Design review of the part built by this model. Coordinates are the model's own, in mm. Face numbers are marked on the shaded views. A direction names the side the tool comes from. Give positions to 0.01 mm unless a question says otherwise; leave off trailing zeros. Order: outer loops, then holes, each group sorted by start corner. A loop starts at its lowest first (then second) coordinate and runs counter-clockwise, first axis right, second up. Notation, with made-up numbers: (76.25, 6) -> (105.25, 6) arc R33 cw to (105.25, 36) -> close; hole circle Ø1 at (51.5, 58.25). An arc over 180 degrees is marked (long way). Return JSON: item names as keys, results as strings.
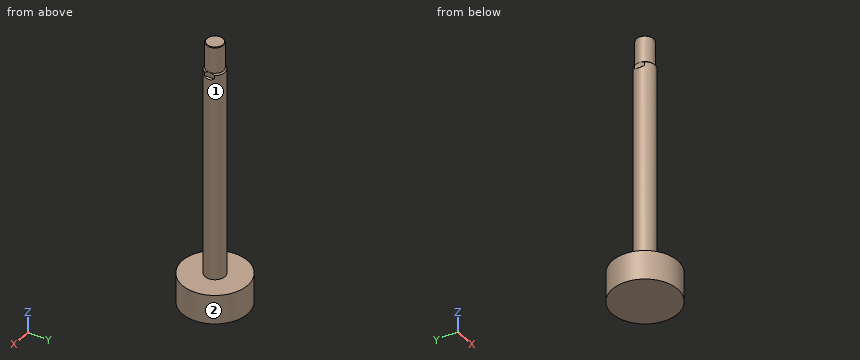
```python
from build123d import *

# Parameters (mm, degrees)
CUT_EXTRUDE_1_DEPTH      = 15
CUT_EXTRUDE_1_DEPTH_BACK = 15
CUT_EXTRUDE_2_DEPTH      = 15
CUT_EXTRUDE_2_DEPTH_BACK = 15


with BuildPart() as part:
    # Sketch 1 → Revolve 1 (revolve)
    with BuildSketch(Plane(origin=(0, 0, 0), x_dir=(0, 0, -1), z_dir=(1, 0, 0))):
        Polygon((-52, 0), (-52, 12.08), (-51.08, 13), (-12, 13), (-10, 15), (305, 15), (305, 49.5), (349, 49.5), (349, 0), align=None)
    revolve(axis=Axis((0, 0, -349), (0, 0, 1)))

    # Sketch 2 → Cut-Extrude 1 (cut, two sides)
    with BuildSketch(Plane(origin=(0, 0, 0), x_dir=(1, 0, 0), z_dir=(0, 1, 0))) as cut_extrude_1_sk:
        Polygon((13, -4.4), (13, -12), (15, -12), (15, -2.4), align=None)
    extrude(amount=CUT_EXTRUDE_1_DEPTH, mode=Mode.SUBTRACT)
    extrude(cut_extrude_1_sk.sketch, amount=-CUT_EXTRUDE_1_DEPTH_BACK, mode=Mode.SUBTRACT)

    # Sketch 3 → Cut-Extrude 2 (cut, two sides)
    with BuildSketch(Plane(origin=(0, 0, 0), x_dir=(1, 0, 0), z_dir=(0, 1, 0))) as cut_extrude_2_sk:
        Polygon((-15, -2.4), (-15, -12), (-13, -12), (-13, -4.4), align=None)
    extrude(amount=CUT_EXTRUDE_2_DEPTH, mode=Mode.SUBTRACT)
    extrude(cut_extrude_2_sk.sketch, amount=-CUT_EXTRUDE_2_DEPTH_BACK, mode=Mode.SUBTRACT)


solid = part.part
```
Item 1: For pin 1 (2.5 mm diameter, centred on y = -0.5, z = 9.5, fed in from -X); pin 2 (6 mm diameter, centred on y = 0.5, z = 7, fed in from +X); pin 3 (10 mm diameter, centred on x = -11, z = -140.5, fed in from +Y), all flat-tipped, find the tip position at first contact; note any pin that passes through.
Result set:
{"pin 1": "stops at x = -13", "pin 2": "stops at x = 13.4", "pin 3": "stops at y = 13.75"}
Item 2: Wall thickness on L1, parallel to Y at x = -1, z = -61.5; L2, parallel to Z at x = -6, y = 33.5; L3, parallel to Y at x = 9, z = -90: over which ranges is each line inside the solid? List them lowest first. Write a range as [from, to].
Result set:
{"L1": "y = [-14.97, 14.97]", "L2": "z = [-349, -305]", "L3": "y = [-12, 12]"}
Item 3: Add section B-B (z = -103). Give the boundary of the cut face in (x, y), plus the area to 3 significant figures.
Result set:
{"outline": "circle Ø30 at (0, 0)", "area": "707 mm^2"}
Item 4: Machinability: for the marked faces 1 and 2, which of the approach directions +Z, -Z, +X, -X, +Y, -Y give a long, thin tool a straight path to every point of the face, cutting with its end or side? Answer none if there is none.
Result set:
{"face 1": "+Z", "face 2": "+Z, -Z"}
Item 5: Add section D-D (x = -40). Give the boundary of the cut face in (y, z).
Result set:
{"outline": "(-29.16, -349) -> (29.16, -349) -> (29.16, -305) -> (-29.16, -305) -> close"}
Item 6: Add section C-C (y = -27). Give the boundary of the cut face in (x, z), plus the area to 3 significant figures.
Result set:
{"outline": "(-41.49, -349) -> (41.49, -349) -> (41.49, -305) -> (-41.49, -305) -> close", "area": "3,650 mm^2"}
Item 7: Add section A-A (x = 0). Give the boundary of the cut face in (y, z).
Result set:
{"outline": "(-49.5, -349) -> (49.5, -349) -> (49.5, -305) -> (15, -305) -> (15, 10) -> (13, 12) -> (13, 51.08) -> (12.08, 52) -> (-12.08, 52) -> (-13, 51.08) -> (-13, 12) -> (-15, 10) -> (-15, -305) -> (-49.5, -305) -> close"}
